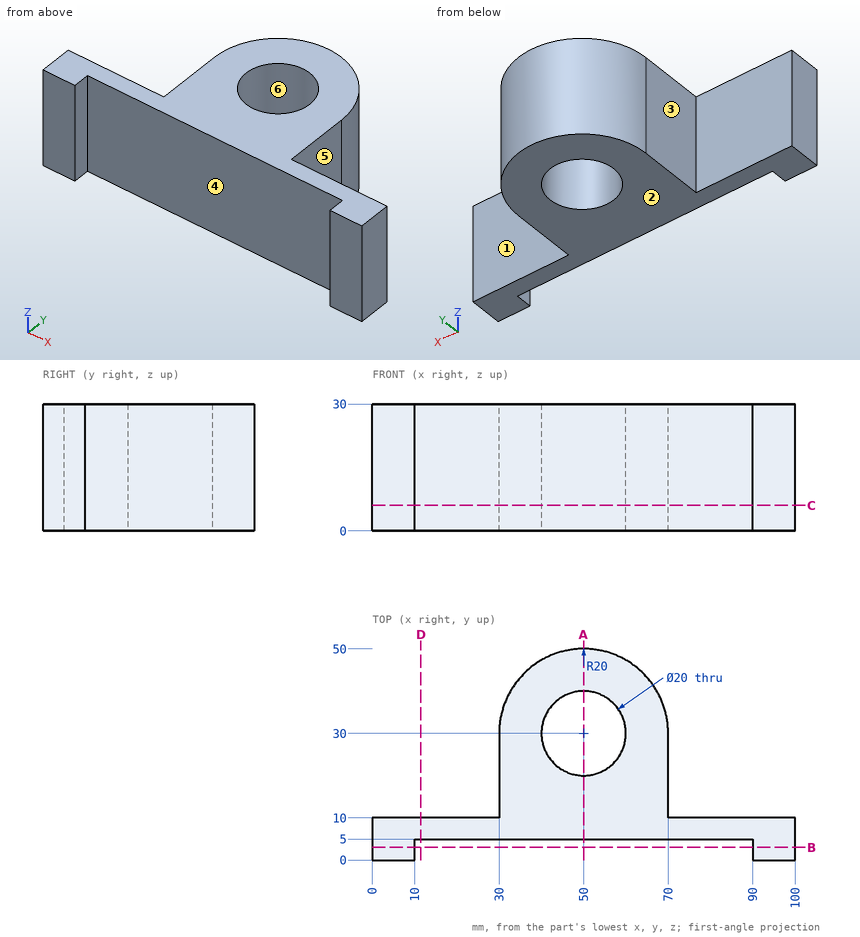
Design review of the part shown in the three views and the two pictorial views. Dimensions are in mm from the part's minimum x, y and z. A direction names the side the tool comes from. Coordinates: 2 decimals unless noted, no trailing zeros. Order: outer loops, then holes, each group sorted by start corner. A loop starts at its lowest first (then second) coordinate and runs counter-clockwise, first axis right, second up.
1) Take a section at A-A, the plane x = 50. Give the boundary of the cut face in (y, z).
2) Clearance check with flat-ended pins moving along their axes: pin 1 (10 mm diameter, centred on y = 18, z = 18, fed in from +X); pin 2 (10 mm diameter, centred on y = 32, z = 20, fed in from -X); pin 3 (2 mm diameter, centred on x = 28, z = 23.5, fed in from -Y). State where each tip first meets the part, or that it passes through.
3) Take a section at B-B, the plane y = 3. Give the boundary of the cut face in (x, z).
4) Take a section at C-C, the plane z = 6. Give the boundary of the cut face in (x, y).
5) Wall thickness on line 1 along Y through (x, z) = (50, 18.75); line 2 along Y through (x, z) = (41, 7.5); line 3 along Y through (x, z) = (76.5, 25.5): over which ranges is each line inside the solid? List them lowest first.
6) Mouldability with a two-part tool opening along Y and no side actions: class the marked faces 4, 5 and 6 as +Y half, -Y half, draft (parallel to the pull), parting line (faces both ways), or undercut.
7) Take a section at D-D, the plane x = 11.5. Give the boundary of the cut face in (y, z).
8) For the marked faces 1, 2 and 3, list the 3-axis set-ups (+Z, -Z, +X, -X, +Y, -Y) from which the entire face can be reached by the end or side of a thin tool; tool diameter is ignored.
Returned:
1. outline: (5, 0) - (20, 0) - (20, 30) - (5, 30) - close; (40, 0) - (50, 0) - (50, 30) - (40, 30) - close
2. pin 1: stops at x = 70
2. pin 2: stops at x = 30
2. pin 3: stops at y = 5
3. outline: (0, 0) - (10, 0) - (10, 30) - (0, 30) - close; (90, 0) - (100, 0) - (100, 30) - (90, 30) - close
4. outline: (0, 0) - (10, 0) - (10, 5) - (90, 5) - (90, 0) - (100, 0) - (100, 10) - (70, 10) - (70, 30) arc R20 ccw to (30, 30) - (30, 10) - (0, 10) - close; hole circle Ø20 at (50, 30)
5. line 1: y = 5 to 20, 40 to 50
5. line 2: y = 5 to 25.64, 34.36 to 47.86
5. line 3: y = 5 to 10
6. face 4: -Y half
6. face 5: draft
6. face 6: undercut
7. outline: (5, 0) - (10, 0) - (10, 30) - (5, 30) - close
8. face 1: +Z, -Z, +X, +Y
8. face 2: -Z, +X, -X, +Y, -Y
8. face 3: +Z, -Z, -X, +Y
